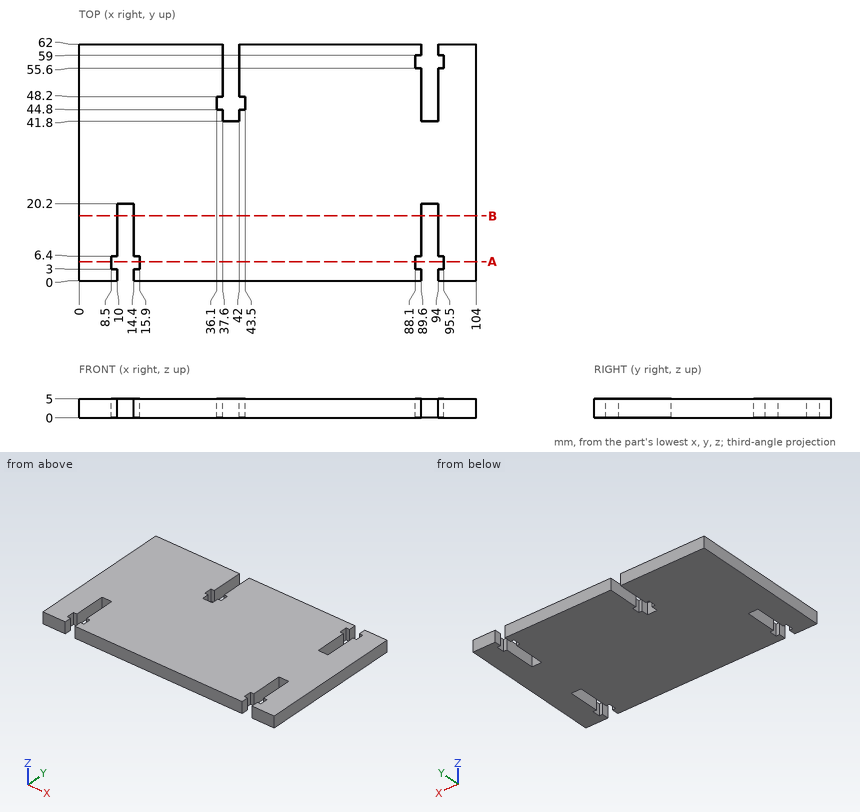
Here's the drawing with two shaded views (mm, measured from the low corner). I have some questions. Coordinates: 2 decimals unless noted, no trailing zeros. Loops run counter-clockwise (first coordinate to the right, second up) from the corner with the lowest first, then second, coordinate; pieces in that order, holes last.
Item 1: Please list where these lines run through material, in increasing order: L1, parallel to X at y = 50, z = 0.5; L2, parallel to X at y = 5, z = 3.4.
Answers below:
L1: x = 0 to 37.6, 42 to 89.6, 94 to 104
L2: x = 0 to 8.5, 15.9 to 88.1, 95.5 to 104
Item 2: I'm going to push flat-ended pins straight in: pin 1 (1.3 mm diameter, centred on x = 11.5, z = 1.5, fed in from -Y); pin 2 (1.3 mm diameter, centred on x = 39.5, z = 3, fed in from +Y). Where does each tip first touch, or does it pass through?
Answers below:
pin 1: stops at y = 20.2
pin 2: stops at y = 41.8
Item 3: Suppose I cut it at B-B (y = 17). Please give me the cut outline in (x, z).
Answers below:
outline: (0, 0) - (10, 0) - (10, 5) - (0, 5) - close; (14.4, 0) - (89.6, 0) - (89.6, 5) - (14.4, 5) - close; (94, 0) - (104, 0) - (104, 5) - (94, 5) - close
Item 4: Suppose I cut it at A-A (y = 5). Please give me the cut outline in (x, z).
Answers below:
outline: (0, 0) - (8.5, 0) - (8.5, 5) - (0, 5) - close; (15.9, 0) - (88.1, 0) - (88.1, 5) - (15.9, 5) - close; (95.5, 0) - (104, 0) - (104, 5) - (95.5, 5) - close
